Input: part model. Units: mm. Frame: model coordinates. A direction names the side the tool comes from. Give positions to 0.01 mm unless a question says otherwise; leave off trailing zeros. Write each loop counter-clockwise with the first axis right and the second up, starting at its lowest first coordinate (ties: lowest second). Pieces come first, ordered by that corner, then holes. Notation, with made-up numbers: (85, 25.25) -> (91, 25.25) arc R26 cw to (91, 55.25) -> close; hole circle Ø8 at (-36, -18). An arc over 180 degrees is marked (long way). Answer as a JSON object with one key per item and string values. Group by question number.
from build123d import *

# Parameters (mm, degrees)
EXTRUDE_1_DEPTH = 1.6
FILLET_1_R      = 1


with BuildPart() as part:
    # 草图1 → 凸台-拉伸1 (new body)
    with BuildSketch(Plane.XY):
        with BuildLine():
            Line((-0.5, 8.5), (7, 8.5))
            Line((7, 8.5), (7, 13.5))
            Line((7, 13.5), (15, 13.5))
            Line((15, 13.5), (15, -17))
            Line((15, -17), (7, -17))
            Line((7, -17), (7, -8.5))
            Line((7, -8.5), (-0.5, -8.5))
            ThreePointArc((-0.5, -8.5), (-9, 0), (-0.5, 8.5))
        make_face()
        with BuildLine():
            Line((-0.5, 3), (3.5, 3))
            ThreePointArc((3.5, 3), (6.5, 0), (3.5, -3))
            Line((3.5, -3), (-0.5, -3))
            ThreePointArc((-0.5, -3), (-3.5, 0), (-0.5, 3))
        make_face(mode=Mode.SUBTRACT)
        with BuildLine():
            Line((-0.5, 6.75), (3.5, 6.75))
            ThreePointArc((3.5, 6.75), (4.5, 5.75), (3.5, 4.75))
            Line((3.5, 4.75), (-0.5, 4.75))
            ThreePointArc((-0.5, 4.75), (-1.5, 5.75), (-0.5, 6.75))
        make_face(mode=Mode.SUBTRACT)
        with BuildLine():
            Line((-0.5, -6.75), (3.5, -6.75))
            ThreePointArc((3.5, -6.75), (4.5, -5.75), (3.5, -4.75))
            Line((3.5, -4.75), (-0.5, -4.75))
            ThreePointArc((-0.5, -4.75), (-1.5, -5.75), (-0.5, -6.75))
        make_face(mode=Mode.SUBTRACT)
        with BuildLine():
            Line((12.5, -8.5), (12.5, -14.5))
            ThreePointArc((12.5, -14.5), (11, -16), (9.5, -14.5))
            Line((9.5, -14.5), (9.5, -8.5))
            ThreePointArc((9.5, -8.5), (11, -7), (12.5, -8.5))
        make_face(mode=Mode.SUBTRACT)
        with BuildLine():
            Line((12.5, 5), (12.5, 11))
            ThreePointArc((12.5, 11), (11, 12.5), (9.5, 11))
            Line((9.5, 11), (9.5, 5))
            ThreePointArc((9.5, 5), (11, 3.5), (12.5, 5))
        make_face(mode=Mode.SUBTRACT)
    extrude(amount=EXTRUDE_1_DEPTH)

    # 圆角1
    fillet_1_edges = [part.edges().sort_by_distance(p)[0] for p in [
        (7, 8.5, 0.8),
        (7, 13.5, 0.8),
        (15, 13.5, 0.8),
        (15, -17, 0.8),
        (7, -17, 0.8),
        (7, -8.5, 0.8),
    ]]
    fillet(fillet_1_edges, radius=FILLET_1_R)


solid = part.part
1. Line query: line 1 (Y direction, x = 3.25, z = 0.25); line 2 (Y direction, x = 4.25, z = 0.6); line 3 (Y direction, x = 12.25, z = 1.45). Output: solid intervals per line, ascending.
2. Mould query, pull axis Y, two halves, no side actions, for faces 1 (the face through (2, -3, 1)), 2 (the face through (7.285, 13.199, 0.811)), 3 (the face through (14.715, -16.699, 0.811)). Classes: pulls with the +Y half, pulls with the -Y half, needs draft (parallel to the pull), parting line crosses it, or undercut.
3. Section D-D (x = -2). Return the cut outline in (y, z).
4. Section A-A (x = 3). Return the cut outline in (y, z).
5. Section C-C (z = 0.75). State how many separate pieces and enclosed holes the cut face has, plus the area to 3 significant figures.
6. Reachability of faces 4 (the face through (3, -8.5, 1)), 5 (the face through (2, -4.75, 1)), 6 (the face through (7, 11, 1)), 7 (the face through (14.699, 13.215, 0.811)) from +Z, -Z, +X, -X, +Y, -Y: full face, straight path, thin tool, end or side. Return the list, or none.
7. Section B-B (y = -11). Return the cut outline in (x, z).
8. Contact query for flat-ended pins moving along their axis: pin 1 Ø0.8 at (y, z) = (10.5, 1) entering from -X; pin 2 Ø0.5 at (x, z) = (1, 0.5) entering from -Y; pin 3 Ø0.8 at (x, z) = (1, 1) entering from +Y; pin 4 Ø10 at (x, y) = (6, -1) entering from -Z. Output: stop coordinate, or through.
Working result:
{
 "1": {"line 1": "y = -8.5 to -6.75, -4.75 to -3, 3 to 4.75, 6.75 to 8.5", "line 2": "y = -8.5 to -6.41, -5.09 to -2.9, 2.9 to 5.09, 6.41 to 8.5", "line 3": "y = -17 to -15.33, -7.67 to 4.17, 11.83 to 13.5"},
 "2": {"face 1": "undercut", "face 2": "pulls with the +Y half", "face 3": "pulls with the -Y half"},
 "3": {"outline": "(-8.37, 0) -> (-2.6, 0) -> (-2.6, 1.6) -> (-8.37, 1.6) -> close; (2.6, 0) -> (8.37, 0) -> (8.37, 1.6) -> (2.6, 1.6) -> close"},
 "4": {"outline": "(-8.5, 0) -> (-6.75, 0) -> (-6.75, 1.6) -> (-8.5, 1.6) -> close; (-4.75, 0) -> (-3, 0) -> (-3, 1.6) -> (-4.75, 1.6) -> close; (3, 0) -> (4.75, 0) -> (4.75, 1.6) -> (3, 1.6) -> close; (6.75, 0) -> (8.5, 0) -> (8.5, 1.6) -> (6.75, 1.6) -> close"},
 "5": {"separate pieces": "1", "enclosed holes": "5", "area": "360 mm^2"},
 "6": {"face 4": "+Z, -Z, -X, -Y", "face 5": "+Z, -Z", "face 6": "+Z, -Z, -X, +Y", "face 7": "+Z, -Z, +X, +Y"},
 "7": {"outline": "(7, 0) -> (9.5, 0) -> (9.5, 1.6) -> (7, 1.6) -> close; (12.5, 0) -> (15, 0) -> (15, 1.6) -> (12.5, 1.6) -> close"},
 "8": {"pin 1": "stops at x = 7", "pin 2": "stops at y = -8.5", "pin 3": "stops at y = 8.5", "pin 4": "stops at z = 0"}
}
